Can you work these out from the drawing? Everything is in mm from the part's minimum corner. Round coordinates to 2 decimals unless told otherwise and drop trailing zeros. Order: outer loops, then holes, each group sorted by start corner. A loop starts at its lowest first (then second) coordinate and runs counter-clockwise, first axis right, second up. Notation, with made-up numbers: M 48.5,48.5 L 68.5,48.5 A34 cw 68.5,78.5 Z; hole C 39.5,13.25 d6. An arc over 180 degrees is marked long. Answer as a JSON object with one key per item and string values. Group by question number.
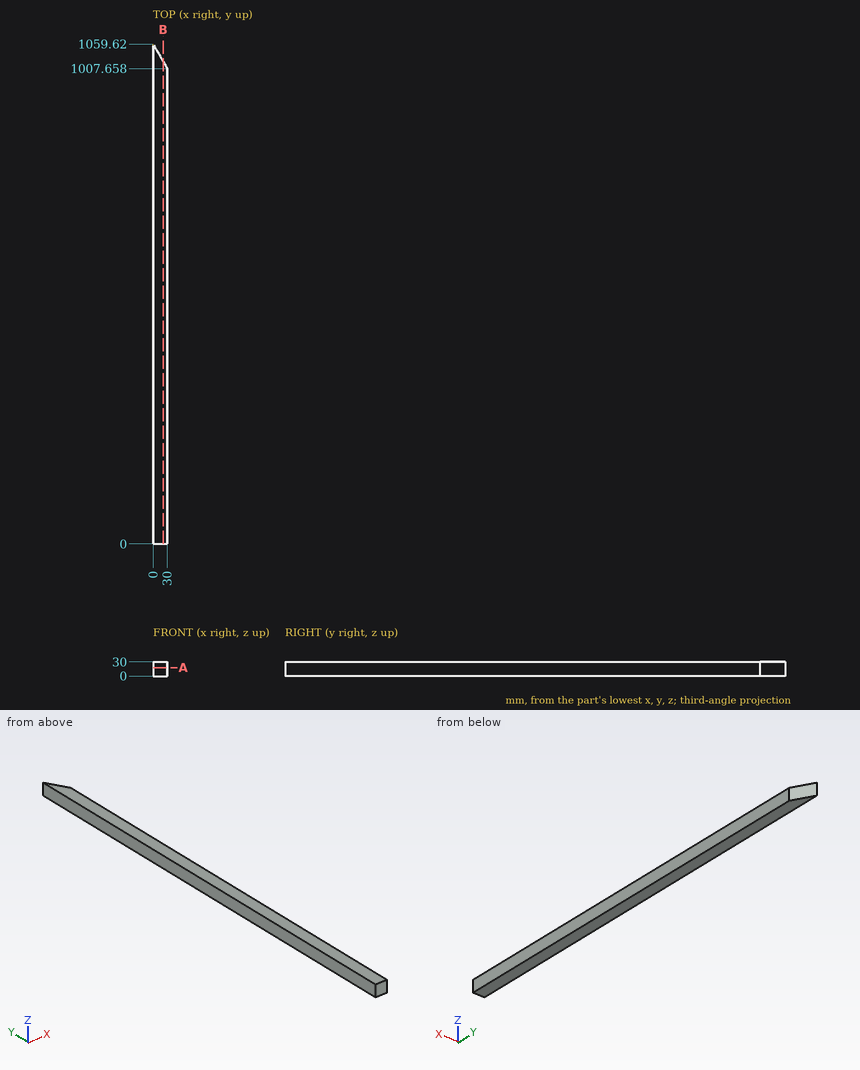
Item 1: Suppose I cut it at B-B, the plane x = 21.25. Write out the boundary of the cut face in (y, z), and give its area (3 significant figures).
Item 2: Suppose I cut it at A-A, the plane z = 18. Write out the boundary of the cut face in (x, y), and give its area (3 significant figures).
Item 3: I need wall thicknesses on line 1 (Y direction, x = 26, z = 24.5) (1 decimal); line 2 (Y direction, x = 4, z = 8.75) (1 decimal). Which ranges of each line are inside material? Lowest first, please.
Computed:
{
 "1": {"outline": "M 0,0 L 1022.81,0 L 1022.81,30 L 0,30 Z", "area": "30,700 mm^2"},
 "2": {"outline": "M 0,0 L 30,0 L 30,1007.66 L 0,1059.62 Z", "area": "31,000 mm^2"},
 "3": {"line 1": "y = 0 to 1014.6", "line 2": "y = 0 to 1052.7"}
}
